Input: part model. Units: mm. Frame: model coordinates. A direction names the side the tool comes from. Round coordinates to 2 decimals unless told otherwise and drop trailing zeros. Loops run counter-clockwise (first coordinate to the right, second up) from the corner with the lowest first, then second, coordinate; pieces in that order, holes last.
(1) Access query for faces 1 (the face through (7, -2, 6)), 2 (the face through (0.99, 5.86, 5.36)), 3 (the face through (7, 0, 3)), 4 (the face through (9, 4.5, 4)). Directions: +Z, -Z, +X, -X, +Y, -Y. A direction counts if a zero-diameter tool reaches every point of the face in a straight line with its end or side. Return the directions, or none.
(2) Cut plane C-C, the plane z = 3.75. Give the number of separate pieces and of enclosed holes in the cut face, and give its area (3 significant figures).
(3) Cut plane B-B, the plane z = 7.25. Output: boundary loops of the cut face in (x, y).
(4) First-contact query: pin 1 Ø3 at (x, z) = (12, 6) entering from +Y; pin 2 Ø1.5 at (x, y) = (7, 9) entering from -Z; pin 3 Ø0.7 at (x, y) = (8, 1) entering from -Z. Flat tips, straight axial feed; report the tip coordinate or a pass-through.
(5) Cut plane D-D, the plane y = 11. Output: boundary loops of the cut face in (x, z), and give its area (3 significant figures).
(6) Draft query along Z for faces 5 (the face through (4, 5, 0)), 6 (the face through (1, 8, 6.75)), 7 (the face through (14, 2, 6)). Return one class per face: released by +Z, released by -Z, zero draft, split by the parting line, or undercut.
(7) Cut plane A-A, the plane y = 8.25. Output: boundary loops of the cut face in (x, z).
(8) Line query: line 1 (Y direction, x = 2.9, z = 4); line 2 (Y direction, x = 6.75, z = 2.25); line 3 (Y direction, x = 3.65, z = 4). Output: solid intervals per line, ascending.
from build123d import *

# Parameters (mm, degrees)
SKETCH3_W           = 14
SKETCH3_H           = 6.5
BOSS_EXTRUDE2_DEPTH = 8
CUT_EXTRUDE1_DEPTH  = 6
LPATTERN2_COUNT     = 7
LPATTERN2_PITCH     = 2
SKETCH4_W           = 8
SKETCH4_H           = 7.5
BOSS_EXTRUDE3_DEPTH = 5
CUT_EXTRUDE2_DEPTH  = 2
SKETCH6_R           = 1.6
CUT_EXTRUDE3_DEPTH  = 10
BOSS_EXTRUDE4_DEPTH = 4


with BuildPart() as part:
    # Sketch3 → Boss-Extrude2 (new body)
    with BuildSketch(Plane.XY):
        with Locations((7, 1.25)):
            Rectangle(SKETCH3_W, SKETCH3_H)
    extrude(amount=BOSS_EXTRUDE2_DEPTH)

    # Sketch1 → Cut-Extrude1 (cut)
    with BuildSketch(Plane.XY):
        with BuildLine():
            Line((0.740175425, 0.63), (1.259824575, 0.63))
            ThreePointArc((1.259824575, 0.63), (1.358731646, 0.667228588), (1.408543109, 0.760434783))
            ThreePointArc((1.408543109, 0.760434783), (1.442388286, 0.918062154), (1.501123596, 1.068202247))
            ThreePointArc((1.501123596, 1.068202247), (1.705850588, 1.295639059), (2, 1.38))
            Line((2, 1.38), (2, 0))
            Line((2, 0), (0, 0))
            Line((0, 0), (0, 1.38))
            ThreePointArc((0, 1.38), (0.294149412, 1.295639059), (0.498876404, 1.068202247))
            ThreePointArc((0.498876404, 1.068202247), (0.557611714, 0.918062154), (0.591456891, 0.760434783))
            ThreePointArc((0.591456891, 0.760434783), (0.641268354, 0.667228588), (0.740175425, 0.63))
        make_face()
    cut_extrude1 = extrude(amount=CUT_EXTRUDE1_DEPTH, mode=Mode.SUBTRACT)

    # LPattern2: Cut-Extrude1 ×7
    with Locations(*[(i * LPATTERN2_PITCH, 0, 0) for i in range(1, LPATTERN2_COUNT)]):
        add(cut_extrude1, mode=Mode.SUBTRACT)

    # Sketch4 → Boss-Extrude3 (add)
    with BuildSketch(Plane.ZY):
        with Locations((4, 8.25)):
            Rectangle(SKETCH4_W, SKETCH4_H)
    extrude(amount=-BOSS_EXTRUDE3_DEPTH)

    # Sketch5 → Cut-Extrude2 (cut)
    with BuildSketch(Plane.ZY):
        Polygon((1.25, 9.83771324), (1.25, 6.66228676), (4, 5.074573519), (6.75, 6.66228676), (6.75, 9.83771324), (4, 11.425426481), align=None)
    extrude(amount=-CUT_EXTRUDE2_DEPTH, mode=Mode.SUBTRACT)

    # Sketch6 → Cut-Extrude3 (cut)
    with BuildSketch(Plane.ZY.offset(-2)):
        with Locations((4, 8.25)):
            Circle(SKETCH6_R)
    extrude(amount=-CUT_EXTRUDE3_DEPTH, mode=Mode.SUBTRACT)

    # Sketch7 → Boss-Extrude4 (add)
    with BuildSketch(Plane.XY.offset(8)):
        Polygon((14, -2), (14, 4.5), (5, 12), (0, 12), (0, -2), align=None)
    extrude(amount=BOSS_EXTRUDE4_DEPTH)


solid = part.part
Reported:
1. face 1: +Z, -Z, +X, -X, -Y
1. face 2: -X
1. face 3: -Z, +X, -X
1. face 4: -Z, +X, +Y
2. separate pieces: 3
2. enclosed holes: 0
2. area: 93.0 mm2
3. outline: (0, -2) - (14, -2) - (14, 4.5) - (5, 4.5) - (5, 12) - (0, 12) - close
4. pin 1: stops at y = 4.5
4. pin 2: stops at z = 8
4. pin 3: stops at z = 6
5. outline: (0, 0) - (5, 0) - (5, 8) - (6.2, 8) - (6.2, 12) - (0, 12) - (0, 4.74) - (2, 4.74) - (2, 3.26) - (0, 3.26) - close
5. area: 61.9 mm2
6. face 5: released by -Z
6. face 6: undercut
6. face 7: zero draft
7. outline: (0, 0) - (5, 0) - (5, 2.4) - (2, 2.4) - (2, 1.25) - (0, 1.25) - close; (0, 6.75) - (2, 6.75) - (2, 5.6) - (5, 5.6) - (5, 8) - (9.5, 8) - (9.5, 12) - (0, 12) - close
8. line 1: y = -2 to 0, 0.63 to 6.65, 9.85 to 12
8. line 2: y = -2 to 0, 0.63 to 4.5
8. line 3: y = -2 to 0, 1.26 to 6.65, 9.85 to 12
